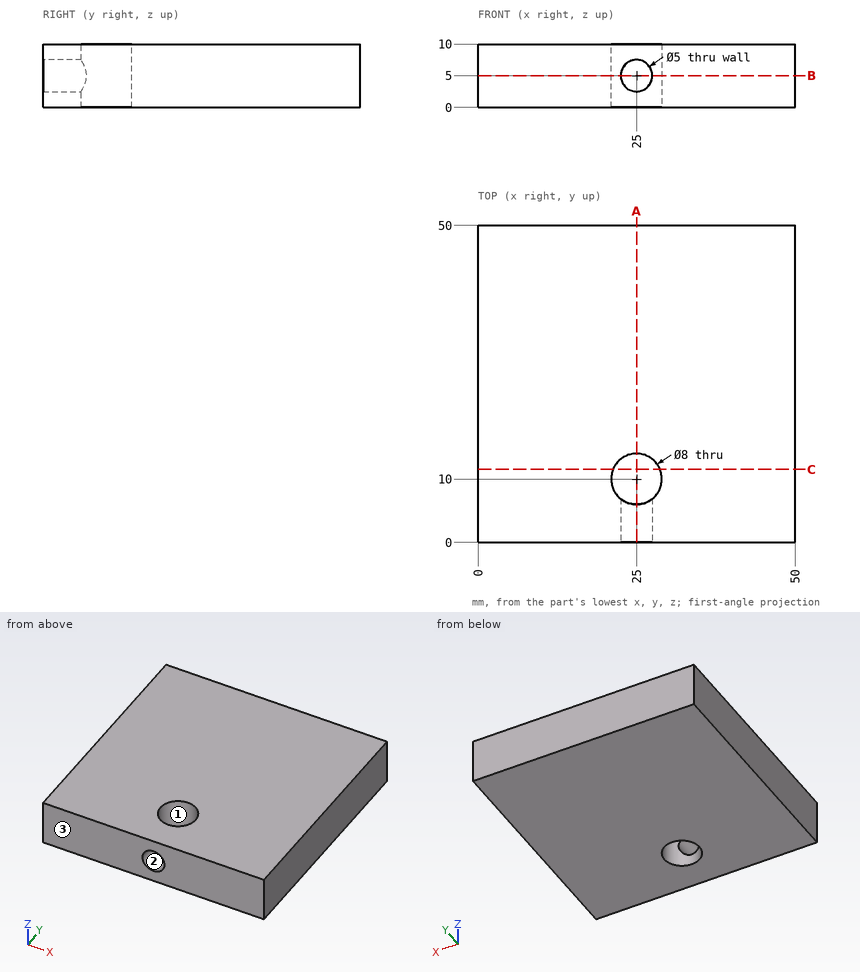
Part print with two shaded views. Sizes in mm from the minimum x, y, z corner. Coordinates: 2 decimals unless noted, no trailing zeros. Order: outer loops, then holes, each group sorted by start corner. A loop starts at its lowest first (then second) coordinate and runs counter-clockwise, first axis right, second up. Notation, with made-up numbers: M 41,28.25 L 53,28.25 A17 cw 53,49.25 Z; hole C 60,-29.75 d1. An arc over 180 degrees is marked long. Use a Markdown table: item, result.
(1) Probe L1, parallel to Z at x = 25, y = 4.5; L2, parallel to X at y = 3.5, z = 5; L3, parallel to Y at x = 25, z = 7. List the from-to ranges inside material, lowest first.
A:
| item | result |
|---|---|
| L1 | z = 0 to 2.5, 7.5 to 10 |
| L2 | x = 0 to 22.5, 27.5 to 50 |
| L3 | y = 14 to 50 |
(2) Cut at B-B on z = 5. Write the cut outline in (x, y), then the cut area to 3 significant figures.
A:
| item | result |
|---|---|
| outline | M 0,0 L 22.5,0 L 22.5,6.88 A4 cw long 27.5,6.88 L 27.5,0 L 50,0 L 50,50 L 0,50 Z |
| area | 2,420 mm^2 |
(3) Cut at A-A on x = 25. Write the cut outline in (y, z).
A:
| item | result |
|---|---|
| outline | M 0,0 L 6,0 L 6,2.5 L 0,2.5 Z; M 0,7.5 L 6,7.5 L 6,10 L 0,10 Z; M 14,0 L 50,0 L 50,10 L 14,10 Z |
(4) Pull direction Y, two halves, no side cores. Call the marked faces 1, 2 and 3: released by +Y, released by -Y, zero draft, split by the parting line, or undercut.
A:
| item | result |
|---|---|
| face 1 | undercut |
| face 2 | zero draft |
| face 3 | released by -Y |
(5) Cut at C-C on y = 11.5. Write the cut outline in (x, z), then the cut area to 3 significant figures.
A:
| item | result |
|---|---|
| outline | M 0,0 L 21.29,0 L 21.29,10 L 0,10 Z; M 28.71,0 L 50,0 L 50,10 L 28.71,10 Z |
| area | 426 mm^2 |
